The drawing under review shows one solid part. Ordinate dimensions are in mm from its lowest x, y, z. A direction names the side the tool comes from. Round coordinates to 2 decimals unless told otherwise and drop trailing zeros. Order: outer loops, then holes, each group sorted by start corner. A loop starts at its lowest first (then second) coordinate and runs counter-clockwise, first axis right, second up. Notation, with made-up numbers: (-16, -25.75) -> (6, -25.75) arc R17 cw to (6, -16.75) -> close; hole circle Ø6 at (48.25, 45.25). An arc over 180 degrees is marked (long way). Return JSON: item names as keys, results as strings. Group by question number.
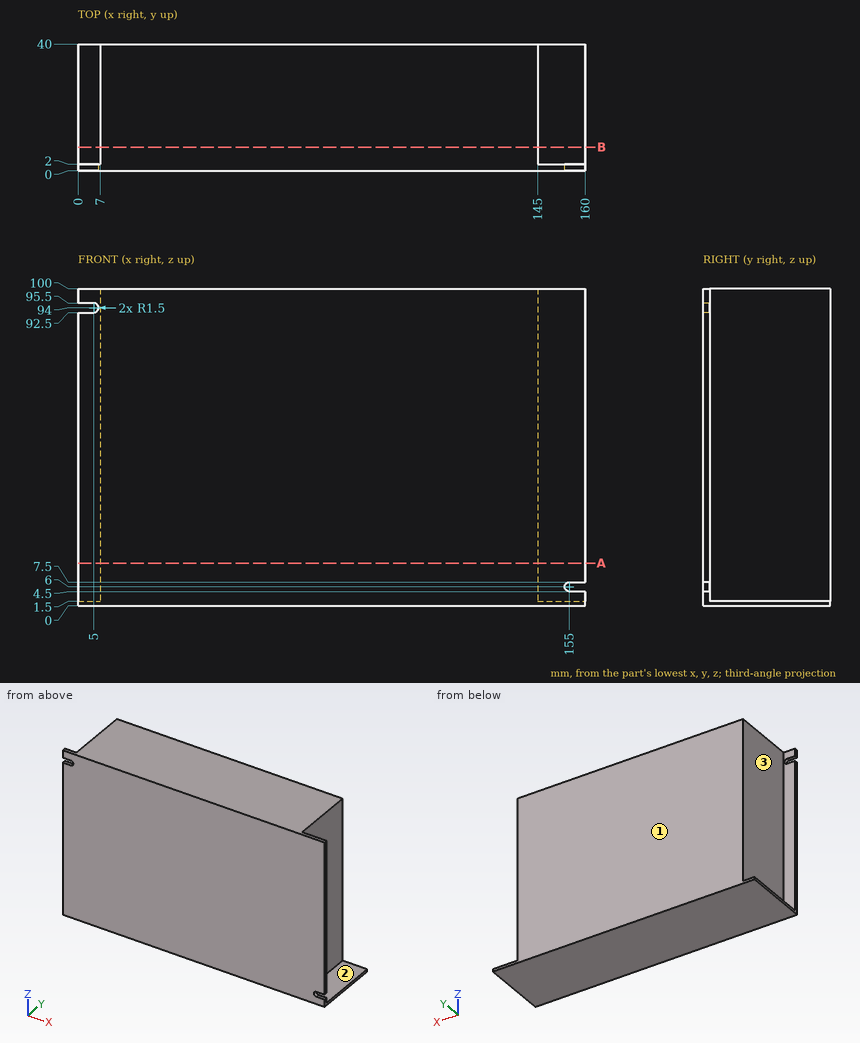
Item 1: Consider section B-B on y = 7.5. State the section outline as (x, z) points, plus the area to 3 significant figures.
Item 2: Insertion check: pin 1 Ø19 at (y, z) = (16, 28.5) entering from -X; pin 2 Ø1 at (y, z) = (15, 69) entering from +X; pin 3 Ø4.5 at (x, y) = (154, 26) entering from +Z. Each pin has a flat end and moves straight along its axis. Give the tip position at first contact, or say it passes through.
Item 3: For the marked faces 1, 2 and 3, list the 3-axis set-ups (+Z, -Z, +X, -X, +Y, -Y) from which the entire face can be reached by the end or side of a thin tool; tool diameter is ignored.
Item 4: Consider section A-A on z = 13.5. State the section outline as (x, y) points.
Item 5: Wall thickness on line 1 along X through (y, z) = (36, 9.5); line 2 along Y through (x, z) = (149.5, 41); line 3 along Z through (x, y) = (149, 26): over which ranges is each line inside the solid? List them lowest first.
Values:
{
 "1": {"outline": "(0, 0) -> (160, 0) -> (160, 1.5) -> (145, 1.5) -> (145, 100) -> (7, 100) -> (7, 1.5) -> (0, 1.5) -> close", "area": "13,800 mm^2"},
 "2": {"pin 1": "x = 7", "pin 2": "x = 145", "pin 3": "z = 1.5"},
 "3": {"face 1": "+Z, -Z, +X, -X, +Y", "face 2": "+Z, +X, +Y", "face 3": "+Z, -X, +Y"},
 "4": {"outline": "(0, 0) -> (160, 0) -> (160, 2) -> (145, 2) -> (145, 40) -> (7, 40) -> (7, 2) -> (0, 2) -> close"},
 "5": {"line 1": "7 to 145", "line 2": "0 to 2", "line 3": "0 to 1.5"}
}
